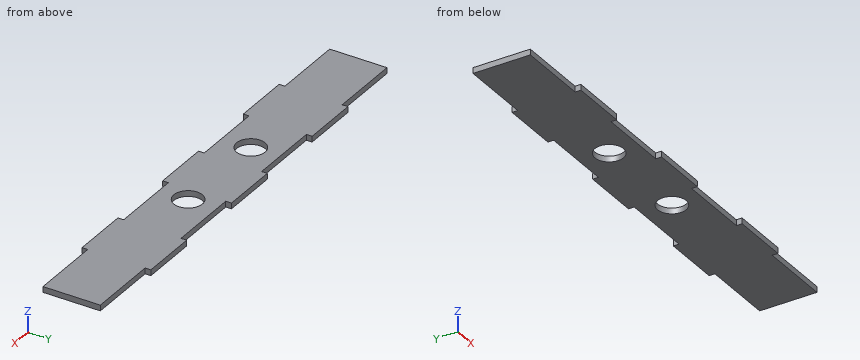
```python
from build123d import *

# Parameters (mm, degrees)
SKETCH_1_R      = 5
EXTRUDE_1_DEPTH = 2


with BuildPart() as part:
    # Эскиз1 → Бобышка-Вытянуть1 (new body)
    with BuildSketch(Plane.XY):
        Polygon((25, 2), (25, 0), (45, 0), (45, 2), (70, 2), (70, 0), (90, 0), (90, 2), (115, 2), (115, 0), (135, 0), (135, 2), (160, 2), (160, 22), (135, 22), (135, 24), (115, 24), (115, 22), (90, 22), (90, 24), (70, 24), (70, 22), (45, 22), (45, 24), (25, 24), (25, 22), (0, 22), (0, 2), align=None)
        with Locations((60, 12)):
            Circle(SKETCH_1_R, mode=Mode.SUBTRACT)
        with Locations((95, 12)):
            Circle(SKETCH_1_R, mode=Mode.SUBTRACT)
    extrude(amount=EXTRUDE_1_DEPTH)


solid = part.part
```
Model file for the job. Use its own axes, mm. Coordinates: 2 decimals unless noted, no trailing zeros. Loops run counter-clockwise (first coordinate to the right, second up) from the corner with the lowest first, then second, coordinate; pieces in that order, holes last. Notation, with made-up numbers: M 22,68.5 L 27,68.5 A24 cw 27,106.5 Z; hole C 24.25,24.25 d1. An arc over 180 degrees is marked long. Use CSV: the item, a comma, the result in double quotes. Start each with the question number.
1. Flat gauge pins, fed straight in: pin 1 (0.6 mm diameter, centred on y = 1.5, z = 0.5, fed in from +X); pin 2 (1 mm diameter, centred on y = 23.5, z = 1.5, fed in from -X); pin 3 (1 mm diameter, centred on x = 97.5, z = 0.5, fed in from +Y); pin 4 (8 mm diameter, centred on x = 60, y = 12, fed in from -Z). Where does each tip first touch, or does it go through?
2. Band-saw the part on A-A, the plane y = 12. List the corners of the cut face in (x, z).
3. Band-saw the part on C-C, the plane x = 60. List the corners of the cut face in (y, z), then the cut area to 3 significant figures.
4. Probe probe 1 along X at (y, z) = (22.5, 1.2); probe 2 along X at (y, z) = (8.5, 1.3); probe 3 along Y at (x, z) = (95, 0.75). List the from-to ranges inside material, lowest first. Write a range as [from, to].
5. Band-saw the part on D-D, the plane x = 113. List the corners of the cut face in (y, z), then the cut area to 3 significant figures.
6. Band-saw the part on B-B, the plane z = 1.35. Give the number of separate pieces and of enclosed holes in the cut face, then the cut area to 3 significant figures.
Entries:
1,pin 1,"stops at x = 135"
1,pin 2,"stops at x = 25"
1,pin 3,"stops at y = 22"
1,pin 4,"passes through"
2,outline,"M 0,0 L 55,0 L 55,2 L 0,2 Z; M 65,0 L 90,0 L 90,2 L 65,2 Z; M 100,0 L 160,0 L 160,2 L 100,2 Z"
3,outline,"M 2,0 L 7,0 L 7,2 L 2,2 Z; M 17,0 L 22,0 L 22,2 L 17,2 Z"
3,area,"20.0 mm2"
4,probe 1,"x = [25, 45], [70, 90], [115, 135]"
4,probe 2,"x = [0, 56.43], [63.57, 91.43], [98.57, 160]"
4,probe 3,"y = [2, 7], [17, 22]"
5,outline,"M 2,0 L 22,0 L 22,2 L 2,2 Z"
5,area,"40.0 mm2"
6,separate pieces,"1"
6,enclosed holes,"2"
6,area,"3,280 mm2"
